Part model, mm, in its own coordinate system. Round coordinates to 2 decimals unless told otherwise and drop trailing zeros. Write each loop counter-clockwise with the first axis right and the second up, starting at its lowest first coordinate (ties: lowest second). Pieces come first, ordered by that corner, then holes.
```python
from build123d import *

# Parameters (mm, degrees)
SKETCH062_R     = 75
PAD043_DEPTH    = 1.6
SKETCH063_W     = 42
SKETCH063_H     = 42
POCKET021_DEPTH = 1.601
SKETCH064_W     = 40
SKETCH064_H     = 130
POCKET022_DEPTH = 1.601


with BuildPart() as part:
    # Sketch062 → Pad043 (new body)
    with BuildSketch(Plane.XY):
        Circle(SKETCH062_R)
    extrude(amount=PAD043_DEPTH)

    # Sketch063 (on Face3 of Pad043) → Pocket021 (cut, through all)
    with BuildSketch(Plane.XY.offset(1.6)):
        Rectangle(SKETCH063_W, SKETCH063_H)
    extrude(amount=-POCKET021_DEPTH, mode=Mode.SUBTRACT)

    # Sketch064 (on Face3 of Pocket021) → Pocket022 (cut, through all)
    with BuildSketch(Plane.XY.offset(1.6)):
        with Locations((-60, 0)):
            Rectangle(SKETCH064_W, SKETCH064_H)
    extrude(amount=-POCKET022_DEPTH, mode=Mode.SUBTRACT)


with BuildPart() as part_1:
    # Body024 placement: moved
    add(part.part.moved(Location((0, 0, 16))))


solid = part_1.part
```
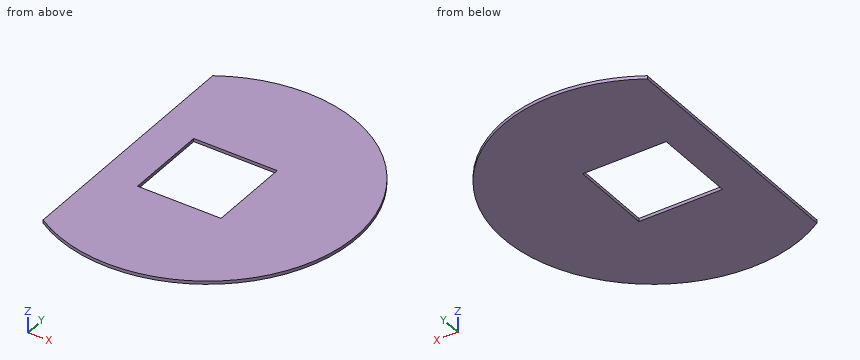
Q1. Cut at D-D on x = 23.5. Write the cut outline in (y, z), plus the area to 3 significant figures.
Values follow:
outline: (-71.22, 16) - (71.22, 16) - (71.22, 17.6) - (-71.22, 17.6) - close
area: 228 mm2
Q2. Wall check: L1, parallel to Y at x = 16.5, z = 16.45; L2, parallel to Y at x = -17, z = 17.5; L3, parallel to X at y = 7.5, z = 16.45. Give the ranges that are in metal, low to high.
Values follow:
L1: y = -73.16 to -21, 21 to 73.16
L2: y = -73.05 to -21, 21 to 73.05
L3: x = -40 to -21, 21 to 74.62
Q3. Cut at B-B on y = 0. Write the cut outline in (x, z), plus the area to 3 significant figures.
Values follow:
outline: (-40, 16) - (-21, 16) - (-21, 17.6) - (-40, 17.6) - close; (21, 16) - (75, 16) - (75, 17.6) - (21, 17.6) - close
area: 117 mm2
Q4. Cut at A-A on x = 0. Write the cut outline in (y, z).
Values follow:
outline: (-75, 16) - (-21, 16) - (-21, 17.6) - (-75, 17.6) - close; (21, 16) - (75, 16) - (75, 17.6) - (21, 17.6) - close
Q5. Cut at C-C on z = 17.1. Write the cut outline in (x, y).
Values follow:
outline: (-40, -63.44) arc R75 ccw (long way) to (-40, 63.44) - close; hole (-21, -21) - (21, -21) - (21, 21) - (-21, 21) - close
Q6. Drop flat-ended pins along their axis: pin 1 (0.5 mm diameter, centred on y = -7.5, z = 16.5, fed in from +X); pin 2 (12 mm diameter, centred on x = 51, y = -57.5, fed in from -Z). Give the stop position or say it passes through.
Values follow:
pin 1: stops at x = 74.65
pin 2: stops at z = 16
